Autodesk Fusion 360 part; units mm, degrees
sketch "Sketch2" plane through (0, 0, 0) normal (0, 0, 1) x (1, 0, 0)
  line L0 (0, 0) -> (0, 65)
  line L1 (13.4496, 0.1022) -> (13.4496, 20.1022)
  line L2 (13.4496, 20.1022) -> (15.9496, 20.1022)
  line L3 (15.9496, 20.1022) -> (15.9496, 28.1022)
  line L4 (15.9496, 28.1022) -> (13.4496, 28.1022)
  line L5 (13.4496, 28.1022) -> (13.4496, 48.1022)
  line L6 (11.4496, 0.1022) -> (11.4496, 22.1022)
  line L7 (11.4496, 22.1022) -> (13.9496, 22.1022)
  line L8 (13.9496, 22.1022) -> (13.9496, 26.1022)
  line L9 (13.9496, 26.1022) -> (11.4496, 26.1022)
  line L10 (11.4496, 26.1022) -> (11.4496, 48.1022)
  line L11 (13.4496, 48.1022) -> (11.4496, 48.1022)
  line L12 (11.4496, 0.1022) -> (13.4496, 0.1022)
  line L13 (11.4496, 26.1022) -> (11.4496, 22.1022)
  line L14 (13.4496, 20.1022) -> (15.9496, 21.6691)
  line L15 (15.9496, 24.1022) -> (11.5, 24.1022)
  line L16 (13.4496, 28.1022) -> (15.9496, 26.5353)
  dimension "d2" = 13.45
  dimension "d3" = 20
  dimension "d4" = 20
  dimension "d5" = 8
  dimension "d6" = 2.5
  dimension "d7" = -2
revolve "Revolve1" add sketch "Sketch2" angle 360 about axis through (0, 0, 0) along (0, 1, 0) contours L1 L3 L6 L7 L8 L12 L14 L15 | L7 L8 L9 L13 | L3 L5 L8 L9 L10 L11 L15 L16
equation "d2 = ( 26.9 / 2 ) * 1 mm"
equation "d4 = d3"
CAD build for the part. Positions are in the model's coordinates, mm. A direction names the side the tool comes from. Coordinates: 2 decimals unless noted, no trailing zeros. Write each loop counter-clockwise with the first axis right and the second up, starting at its lowest first coordinate (ties: lowest second). Pieces come first, ordered by that corner, then holes. Notation, with made-up numbers: M 39.5,-30 L 53.5,-30 A24 ccw 53.5,-19 Z; hole C 77.5,-10.5 d9. An arc over 180 degrees is marked long. Return JSON: item names as keys, results as strings.
Item 1: Probe line 1 (Z direction, x = 0, y = 17); line 2 (Z direction, x = -7, y = 10.5). List the from-to ranges inside material, lowest first. Write a range as from..to.
Findings below:
{"line 1": "z = -13.45..-11.45, 11.45..13.45", "line 2": "z = -11.48..-9.06, 9.06..11.48"}
Item 2: Drop flat-ended pins along their axis: pin 1 Ø3 at (x, y) = (-1.5, 31.5) entering from -Z; pin 2 Ø1 at (y, z) = (7, 9.5) entering from +X; pin 3 Ø5 at (y, z) = (15, -10.5) entering from -X. Give the stop position or say it passes through.
Findings below:
{"pin 1": "stops at z = -13.45", "pin 2": "stops at x = 9.99", "pin 3": "stops at x = -10.81"}
Item 3: Two-plate mould, pull along X, no slides. Class faces 4 (the cylindrical face through (-2.482, 24.438, 11.177)), 5 (the conical face through (-1.771, 28.004, 13.49)), 6 (the flat face through (10, 48.102, -6)): +X half, -X half, draft (parallel to the pull), parting line (faces both ways), or undercut.
Findings below:
{"face 4": "undercut", "face 5": "parting line", "face 6": "draft"}
Item 4: Slice it at B-B, the plane x = 0. Write the cut outline in (y, z).
Findings below:
{"outline": "M 0.1,-13.45 L 20.1,-13.45 L 21.67,-15.95 L 26.54,-15.95 L 28.1,-13.45 L 48.1,-13.45 L 48.1,-11.45 L 0.1,-11.45 Z; M 0.1,11.45 L 48.1,11.45 L 48.1,13.45 L 28.1,13.45 L 26.54,15.95 L 21.67,15.95 L 20.1,13.45 L 0.1,13.45 Z"}
Item 5: Which spindle directions (+Z, -Z, +X, -X, +Y, -Y) get a long thin tool onto all of the face, cutting with end or side? Do faces 1 (the cylindrical face through (-9.913, 10.242, -9.09)), 2 (the cylindrical face through (-2.076, 24.136, -15.814)), 3 (the cylindrical face through (-9.913, 38.242, -9.09)). Say none if no direction does.
Findings below:
{"face 1": "-Y", "face 2": "+Y, -Y", "face 3": "+Y"}
Item 6: Slice it at C-C, the plane y = 26. Write the cut outline in (x, z), and give its area (3 significant figures).
Findings below:
{"outline": "C 0,0 d31.9; hole C 0,0 d22.9", "area": "387 mm2"}
Item 7: Slice it at D-D, the plane y = 5. Write the cut outline in (x, z).
Findings below:
{"outline": "C 0,0 d26.9; hole C 0,0 d22.9"}
Item 8: Slice it at A-A, the plane z = 0. Write the cut outline in (x, y).
Findings below:
{"outline": "M -15.95,21.67 L -13.45,20.1 L -13.45,0.1 L -11.45,0.1 L -11.45,48.1 L -13.45,48.1 L -13.45,28.1 L -15.95,26.54 Z; M 11.45,0.1 L 13.45,0.1 L 13.45,20.1 L 15.95,21.67 L 15.95,26.54 L 13.45,28.1 L 13.45,48.1 L 11.45,48.1 Z"}
